Here's how the part is built. I have some questions about the finished solid (model axes, mm). Round coordinates to 2 decimals unless told otherwise and drop trailing zeros. Order: outer loops, then holes, each group sorted by start corner. A loop starts at its lowest first (then second) coordinate and runs counter-clockwise, first axis right, second up. Notation, with made-up numbers: (25, 6) - (61, 6) arc R14 ccw to (61, 13) - close; hole circle Ø2 at (30.25, -16.75). An arc over 180 degrees is marked (long way). One line per item, written item: value.
from build123d import *

# Parameters (mm, degrees)
SKETCH1_W           = 100
SKETCH1_H           = 100
BOSS_EXTRUDE1_DEPTH = 12
CUT_EXTRUDE1_REACH  = 88.856
SKETCH2_R           = 3
CUT_EXTRUDE2_REACH  = 88.856
SKETCH3_R           = 13
CUT_EXTRUDE3_REACH  = 88.856
SKETCH4_R           = 6
CUT_EXTRUDE4_REACH  = 88.856
SKETCH5_R           = 28


with BuildPart() as part:
    # Sketch1 → Boss-Extrude1 (new body)
    with BuildSketch(Plane(origin=(0, 0, 0), x_dir=(1, 0, 0), z_dir=(0, 1, 0))):
        with Locations((0, -20)):
            Rectangle(SKETCH1_W, SKETCH1_H)
    extrude(amount=BOSS_EXTRUDE1_DEPTH)

    # Sketch2 → Cut-Extrude1 (cut, up to next)
    with BuildSketch(Plane(origin=(0, 12, 0), x_dir=(1, 0, 0), z_dir=(0, 1, 0)), mode=Mode.PRIVATE) as cut_extrude1_sk1:
        with Locations(Location((-44, 20, 0), (0, 0, 270))):
            Circle(SKETCH2_R)
    cut_extrude1_tool1 = extrude(cut_extrude1_sk1.sketch, amount=-CUT_EXTRUDE1_REACH, mode=Mode.PRIVATE) & part.part
    # Sketch2 → Cut-Extrude1 (cut, up to next)
    with BuildSketch(Plane(origin=(0, 12, 0), x_dir=(1, 0, 0), z_dir=(0, 1, 0)), mode=Mode.PRIVATE) as cut_extrude1_sk2:
        with Locations(Location((-44, 0, 0), (0, 0, 270))):
            Circle(SKETCH2_R)
    cut_extrude1_tool2 = extrude(cut_extrude1_sk2.sketch, amount=-CUT_EXTRUDE1_REACH, mode=Mode.PRIVATE) & part.part
    # Sketch2 → Cut-Extrude1 (cut, up to next)
    with BuildSketch(Plane(origin=(0, 12, 0), x_dir=(1, 0, 0), z_dir=(0, 1, 0)), mode=Mode.PRIVATE) as cut_extrude1_sk3:
        with Locations(Location((44, 20, 0), (0, 0, 270))):
            Circle(SKETCH2_R)
    cut_extrude1_tool3 = extrude(cut_extrude1_sk3.sketch, amount=-CUT_EXTRUDE1_REACH, mode=Mode.PRIVATE) & part.part
    # Sketch2 → Cut-Extrude1 (cut, up to next)
    with BuildSketch(Plane(origin=(0, 12, 0), x_dir=(1, 0, 0), z_dir=(0, 1, 0)), mode=Mode.PRIVATE) as cut_extrude1_sk4:
        with Locations(Location((44, 0, 0), (0, 0, 270))):
            Circle(SKETCH2_R)
    cut_extrude1_tool4 = extrude(cut_extrude1_sk4.sketch, amount=-CUT_EXTRUDE1_REACH, mode=Mode.PRIVATE) & part.part
    add(cut_extrude1_tool1.solids().sort_by_distance((-44, 12, -20))[0], mode=Mode.SUBTRACT)
    add(cut_extrude1_tool2.solids().sort_by_distance((-44, 12, 0))[0], mode=Mode.SUBTRACT)
    add(cut_extrude1_tool3.solids().sort_by_distance((44, 12, -20))[0], mode=Mode.SUBTRACT)
    add(cut_extrude1_tool4.solids().sort_by_distance((44, 12, 0))[0], mode=Mode.SUBTRACT)

    # Sketch3 → Cut-Extrude2 (cut, up to next)
    with BuildSketch(Plane(origin=(0, 12, 0), x_dir=(1, 0, 0), z_dir=(0, 1, 0)), mode=Mode.PRIVATE) as cut_extrude2_sk1:
        with Locations(Location((0, -20, 0), (0, 0, 270))):
            Circle(SKETCH3_R)
    cut_extrude2_tool1 = extrude(cut_extrude2_sk1.sketch, amount=-CUT_EXTRUDE2_REACH, mode=Mode.PRIVATE) & part.part
    add(cut_extrude2_tool1.solids().sort_by_distance((0, 12, 20))[0], mode=Mode.SUBTRACT)

    # Sketch4 → Cut-Extrude3 (cut, up to next)
    with BuildSketch(Plane(origin=(0, 12, 0), x_dir=(1, 0, 0), z_dir=(0, 1, 0)), mode=Mode.PRIVATE) as cut_extrude3_sk1:
        with Locations(Location((-36, -40, 0), (0, 0, 270))):
            Circle(SKETCH4_R)
    cut_extrude3_tool1 = extrude(cut_extrude3_sk1.sketch, amount=-CUT_EXTRUDE3_REACH, mode=Mode.PRIVATE) & part.part
    # Sketch4 → Cut-Extrude3 (cut, up to next)
    with BuildSketch(Plane(origin=(0, 12, 0), x_dir=(1, 0, 0), z_dir=(0, 1, 0)), mode=Mode.PRIVATE) as cut_extrude3_sk2:
        with Locations(Location((36, -40, 0), (0, 0, 270))):
            Circle(SKETCH4_R)
    cut_extrude3_tool2 = extrude(cut_extrude3_sk2.sketch, amount=-CUT_EXTRUDE3_REACH, mode=Mode.PRIVATE) & part.part
    add(cut_extrude3_tool1.solids().sort_by_distance((-36, 12, 40))[0], mode=Mode.SUBTRACT)
    add(cut_extrude3_tool2.solids().sort_by_distance((36, 12, 40))[0], mode=Mode.SUBTRACT)

    # Sketch5 → Cut-Extrude4 (cut, up to next)
    with BuildSketch(Plane(origin=(0, 12, 0), x_dir=(1, 0, 0), z_dir=(0, 1, 0)), mode=Mode.PRIVATE) as cut_extrude4_sk1:
        with Locations((0, -75)):
            Circle(SKETCH5_R)
    cut_extrude4_tool1 = extrude(cut_extrude4_sk1.sketch, amount=-CUT_EXTRUDE4_REACH, mode=Mode.PRIVATE) & part.part
    add(cut_extrude4_tool1.solids().sort_by_distance((0, 12, 75))[0], mode=Mode.SUBTRACT)


solid = part.part
Q1. If I drill on line 1 along X through (y, z) = (7.5, 0); line 2 along X through (y, z) = (6.5, 40); line 3 along X through (y, z) = (5.5, 20), over which ranges is the centre line in solid material (lowest first)?
Results list:
line 1: -50 to -47, -41 to 41, 47 to 50
line 2: -50 to -42, -30 to 30, 42 to 50
line 3: -50 to -13, 13 to 50
Q2. If we section it at C-C, the plane x = 0: Please give me the cut outline in (y, z), then the cut area to 3 significant figures.
Results list:
outline: (0, -30) - (12, -30) - (12, 7) - (0, 7) - close; (0, 33) - (12, 33) - (12, 47) - (0, 47) - close
area: 612 mm²
Q3. Will this pin go through, and if not, where does the flat tip stop? pin 1 (3.5 mm diameter, centred on x = 44, z = 0, fed in from +Y).
Results list:
pin 1: through
Q4. If we section it at D-D, the plane y = 4.25: Please give me the cut outline in (x, z), then the cut area to 3 significant figures.
Results list:
outline: (-50, -30) - (50, -30) - (50, 70) - (27.55, 70) arc R28 cw to (-27.55, 70) - (-50, 70) - close; hole circle Ø6 at (-44, -20); hole circle Ø6 at (-44, 0); hole circle Ø12 at (-36, 40); hole circle Ø26 at (0, 20); hole circle Ø12 at (36, 40); hole circle Ø6 at (44, -20); hole circle Ø6 at (44, 0)
area: 8,180 mm²
Q5. If we section it at A-A, the plane x = -44: Please give me the cut outline in (y, z), then the cut area to 3 significant figures.
Results list:
outline: (0, -30) - (12, -30) - (12, -23) - (0, -23) - close; (0, -17) - (12, -17) - (12, -3) - (0, -3) - close; (0, 3) - (12, 3) - (12, 70) - (0, 70) - close
area: 1,060 mm²
Q6. If we section it at B-B, the plane z = 0: Please give me the cut outline in (x, y).
Results list:
outline: (-50, 0) - (-47, 0) - (-47, 12) - (-50, 12) - close; (-41, 0) - (41, 0) - (41, 12) - (-41, 12) - close; (47, 0) - (50, 0) - (50, 12) - (47, 12) - close
